Input: dimensioned drawing with shaded views. Units: mm. Origin: part minimum x, y, z. A direction names the side the tool comes from. Coordinates: 2 decimals unless noted, no trailing zeros. Order: outer loops, then holes, each group sorted by start corner. A loop starts at its lowest first (then second) coordinate and runs counter-clockwise, first axis right, second up. Notation, with made-up numbers: (53, 88.5) -> (98, 88.5) arc R27 cw to (98, 121.5) -> close; hole circle Ø3 at (12.25, 23.5). An arc over 180 degrees is marked (long way). Answer as CSV lines item,"result".
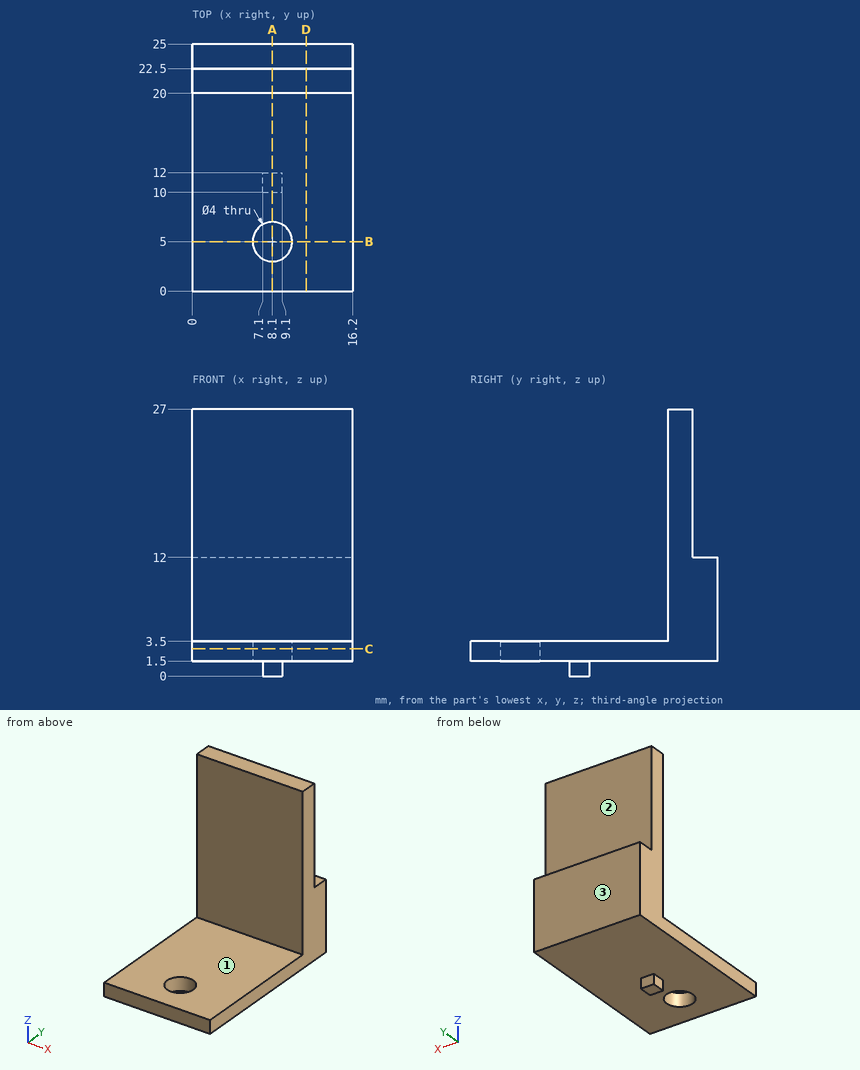
1. Cut plane B-B (y = 5). Return the cut outline in (x, z).
Findings:
outline,"(0, 1.5) -> (6.1, 1.5) -> (6.1, 3.5) -> (0, 3.5) -> close; (10.1, 1.5) -> (16.2, 1.5) -> (16.2, 3.5) -> (10.1, 3.5) -> close"
2. Cut plane A-A (x = 8.1). Return the cut outline in (y, z).
Findings:
outline,"(0, 1.5) -> (3, 1.5) -> (3, 3.5) -> (0, 3.5) -> close; (7, 1.5) -> (10, 1.5) -> (10, 0) -> (12, 0) -> (12, 1.5) -> (25, 1.5) -> (25, 12) -> (22.5, 12) -> (22.5, 27) -> (20, 27) -> (20, 3.5) -> (7, 3.5) -> close"
3. Cut plane C-C (z = 2.75). Return the cut outline in (x, y).
Findings:
outline,"(0, 0) -> (16.2, 0) -> (16.2, 25) -> (0, 25) -> close; hole circle Ø4 at (8.1, 5)"
4. Reachability of the marked faces 1, 2 and 3 from +Z, -Z, +X, -X, +Y, -Y: full face, straight path, thin tool, end or side. Return the list, or none.
Findings:
face 1,"+Z, +X, -X, -Y"
face 2,"+Z, +X, -X, +Y"
face 3,"+Z, -Z, +X, -X, +Y"
5. Contact query for flat-ended pins moving along their axis: pin 1 (6 mm diameter, centred on x = 4, z = 12.5, fed in from -Y); pin 2 (1.5 mm diameter, centred on x = 13.5, y = 8.5, fed in from -Z); pin 3 (6 mm diameter, centred on x = 8.5, y = 11.5, fed in from +Z). Output: stop coordinate, or through.
Findings:
pin 1,"stops at y = 20"
pin 2,"stops at z = 1.5"
pin 3,"stops at z = 3.5"
6. Cut plane D-D (x = 11.5). Return the cut outline in (y, z).
Findings:
outline,"(0, 1.5) -> (25, 1.5) -> (25, 12) -> (22.5, 12) -> (22.5, 27) -> (20, 27) -> (20, 3.5) -> (0, 3.5) -> close"
7. Ray query, line 1 along Y through (x, z) = (8.1, 3.05); line 2 along Z through (x, y) = (6, 11); line 3 along Y through (x, z) = (10.5, 8.25). Return the intervals inside material, ascending.
Findings:
line 1,"y = 0 to 3, 7 to 25"
line 2,"z = 1.5 to 3.5"
line 3,"y = 20 to 25"
